Build history of the part. All positions in model axes, mm. A direction names the side the tool comes from. Coordinates: 2 decimals unless noted, no trailing zeros. Order: outer loops, then holes, each group sorted by start corner. A loop starts at its lowest first (then second) coordinate and runs counter-clockwise, first axis right, second up. Notation, with made-up numbers: (-5, 76.5) - (33, 76.5) arc R16 cw to (33, 96.5) - close; hole circle Ø6 at (28, -12). An arc over 180 degrees is marked (long way). Write each question's results on one line, items separated by ' | '.
from build123d import *

# Parameters (mm, degrees)
F4_R     = 12.875258
F5_DEPTH = 12.7
F6_W     = 8.22093
F6_H     = 18.559195
F7_DEPTH = 25.4
F8_W     = 8.622916
F8_H     = 18.559195
F9_DEPTH = 25.4


with BuildPart() as f1:
    # F0 (on Front) → F1 (revolve)
    with BuildSketch(Plane.XZ):
        Polygon((-34.6094, 4.425088), (-34.6094, -2.110543), (-15.017255, -2.110543), (-15.017255, 46.499304), (-20.429717, 46.499304), (-20.429717, 42.830415), (-24.66305, 42.830415), (-24.66305, 46.499304), (-31.18447, 46.499304), (-31.18447, 34.617999), (-26.812965, 31.212292), (-26.812965, 15.816283), (-31.366523, 10.860938), (-31.366523, 4.425088), align=None)
    revolve(axis=Axis((-15.017255, 0, 22.194381), (0, 0, 1)))


with BuildPart() as f1_1:
    # F2: moved
    add(f1.part.moved(Location((14.986, 0, 2.032))))

    # F4 (on offset) → F5 (cut)
    with BuildSketch(Plane.XY.offset(49.53)):
        Circle(F4_R)
    extrude(amount=-F5_DEPTH, mode=Mode.SUBTRACT)

    # F6 (on Front) → F7 (cut, symmetric)
    with BuildSketch(Plane.XZ):
        with Locations((0, 49.671471)):
            Rectangle(F6_W, F6_H)
    extrude(amount=F7_DEPTH, both=True, mode=Mode.SUBTRACT)

    # F8 (on Right) → F9 (cut, symmetric)
    with BuildSketch(Plane.YZ):
        with Locations((0, 49.528695)):
            Rectangle(F8_W, F8_H)
    extrude(amount=F9_DEPTH, both=True, mode=Mode.SUBTRACT)


solid = f1_1.part
1. Band-saw the part on B-B on y = 0. Give the cut face in (x, z), then the cut area to 3 significant figures.
Solved:
outline: (-19.62, -0.08) - (19.56, -0.08) - (19.56, 6.46) - (16.32, 6.46) - (16.32, 12.89) - (11.76, 17.85) - (11.76, 33.24) - (16.14, 36.65) - (16.14, 40.25) - (12.88, 40.25) - (12.88, 36.83) - (-12.88, 36.83) - (-12.88, 40.25) - (-16.2, 40.25) - (-16.2, 36.65) - (-11.83, 33.24) - (-11.83, 17.85) - (-16.38, 12.89) - (-16.38, 6.46) - (-19.62, 6.46) - close | area: 1,090 mm2
2. Band-saw the part on A-A on z = 43.5. Give the cut face in (x, y), then the cut area to 3 significant figures.
Solved:
outline: (-15.61, -4.31) arc R16.17 ccw to (-4.11, -15.64) - (-4.11, -12.2) arc R12.88 cw to (-12.13, -4.31) - close; (-15.61, 4.31) - (-12.13, 4.31) arc R12.88 cw to (-4.11, 12.2) - (-4.11, 15.64) arc R16.17 ccw to start; (4.11, -15.63) arc R16.17 ccw to (15.55, -4.31) - (12.13, -4.31) arc R12.88 cw to (4.11, -12.2) - close; (4.11, 12.2) arc R12.88 cw to (12.13, 4.31) - (15.55, 4.31) arc R16.17 ccw to (4.11, 15.63) - close | area: 188 mm2
3. Drop flat-ended pins along their axis: pin 1 Ø4.5 at (x, y) = (0.5, -14) entering from +Z; pin 2 Ø4 at (y, z) = (-14.5, 45) entering from +X; pin 3 Ø4.5 at (x, y) = (-13.5, 0) entering from +Z. Give the stop position or say it passes through.
Solved:
pin 1: stops at z = 40.39 | pin 2: stops at x = 10.22 | pin 3: stops at z = 40.25
4. Band-saw the part on C-C on z = 25.5. Give the cut face in (x, y).
Solved:
outline: circle Ø23.59 at (-0.03, 0)
5. Probe line 1 (X direction, y = 0, z = 40); line 2 (Y direction, x = 0.5, z = 29); line 3 (Z direction, x = 9, y = -2). List the from-to ranges inside material, lowest first.
Solved:
line 1: x = -16.2 to -12.88, 12.88 to 16.14 | line 2: y = -11.78 to 11.78 | line 3: z = -0.08 to 36.83
6. Two-plate mould, pull along Z, no slides. Class faces 1 (the face through (0, 14, 40.392)), 2 (the face through (4.11, -14, 44)), 3 (the face through (9.33, 7.18, 25.44)): +Z half, -Z half, draft (parallel to the pull), parting line (faces both ways), or undercut.
Solved:
face 1: +Z half | face 2: draft | face 3: undercut
7. Band-saw the part on D-D on x = 17.5. Give the cut face in (y, z), then the cut area to 3 significant figures.
Solved:
outline: (-8.75, -0.08) - (8.75, -0.08) - (8.75, 6.46) - (-8.75, 6.46) - close | area: 114 mm2
8. Tool access for faces 4 (the face through (-4.11, -14, 44)), 5 (the face through (14, 0, 40.249)), 6 (the face through (0, 0, 36.83)), 7 (the face through (1.5, -11.9, 33.4)): list every direction of +Z, -Z, +X, -X, +Y, -Y with a clear straight run to the whole face (end or side of a thin tool).
Solved:
face 4: +Z, +Y, -Y | face 5: +Z, +X, -X | face 6: +Z | face 7: none
